For this review, use the dimensioned drawing (mm, ordinates from the lowest corner) and the shaded views. Coordinates: 2 decimals unless noted, no trailing zeros. Write each loop counter-clockwise with the first axis right and the second up, starting at its lowest first coordinate (ties: lowest second). Pieces come first, ordered by that corner, then holes. Notation, with made-up numbers: (51.25, -16) - (86.25, -16) arc R16 cw to (86.25, 15) - close; hole circle Ø10 at (73.25, 27). An arc over 180 degrees is marked (long way). One line per item, written item: value.
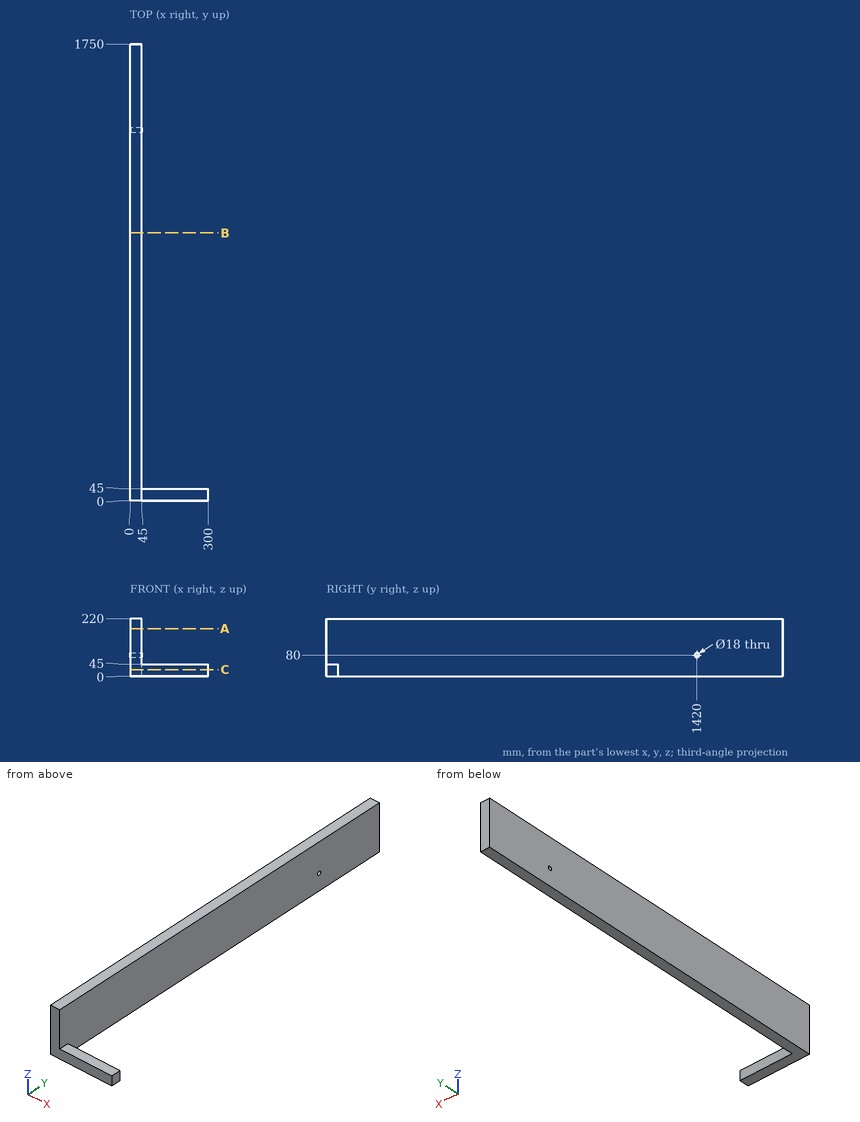
1. Consider section A-A, the plane z = 182. Write out the cut boundary in (x, y).
Answer block:
outline: (0, 0) - (45, 0) - (45, 1750) - (0, 1750) - close
2. Consider section B-B, the plane y = 1026. Write out the cut boundary in (x, z), then the cut area to 3 significant figures.
Answer block:
outline: (0, 0) - (45, 0) - (45, 220) - (0, 220) - close
area: 9,900 mm^2
3. Wall thickness on line 1 along Z through (x, y) = (34.5, 1420); line 2 along X through (y, z) = (212.5, 174.5): over which ranges is each line inside the solid? List them lowest first.
Answer block:
line 1: z = 0 to 71, 89 to 220
line 2: x = 0 to 45
4. Consider section C-C, the plane z = 24. Write out the cut boundary in (x, y), then the cut area to 3 significant figures.
Answer block:
outline: (0, 0) - (300, 0) - (300, 45) - (45, 45) - (45, 1750) - (0, 1750) - close
area: 90,200 mm^2
5. Insertion check: pin 1 Ø8 at (y, z) = (431, 143.5) entering from +X; pin 2 Ø13.5 at (x, y) = (191.5, 25.5) entering from +Z. Each pin has a flat end and moves straight along its axis. Give the tip position at first contact, or say it passes through.
Answer block:
pin 1: stops at x = 45
pin 2: stops at z = 45
